Input: part model. Units: mm. Frame: model coordinates. Face numbers are marked on the shaded views. Round coordinates to 2 decimals unless told otherwise and drop trailing zeros. Write each loop counter-clockwise with the first axis right and the second up, starting at its lowest first coordinate (ties: lowest second). Pieces come first, ordered by that corner, then holes. Notation, with made-up numbers: M 89.5,-16.75 L 99.5,-16.75 A28 ccw 99.5,14.25 Z; hole C -15,-17.75 d6. An arc over 180 degrees is marked long. Answer as CSV lines item,"result". Start each with the question number.
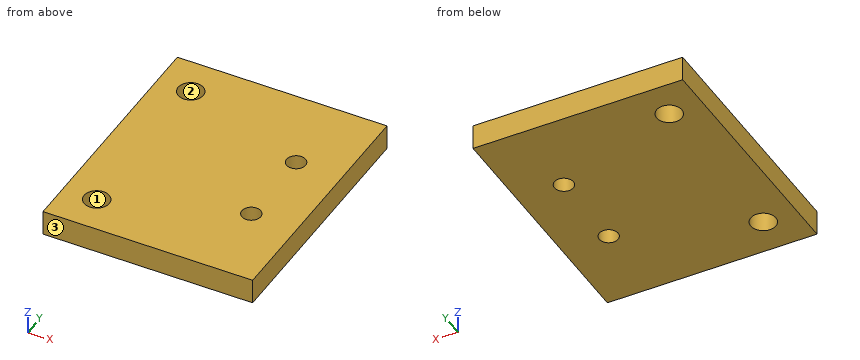
Autodesk Inventor part; units mm, degrees
ref_plane "YZ Plane" through (0, 0, 0) normal (1, 0, 0) x (0, 1, 0)
ref_plane "XZ Plane" through (0, 0, 0) normal (0, 1, 0) x (-1, 0, 0)
ref_plane "XY Plane" through (0, 0, 0) normal (0, 0, 1) x (1, 0, 0)
sketch "Sketch1" plane through (0, 0, 0) normal (0, 0, 1) x (1, 0, 0)
  line L0 (0, 0) -> (50, 0)
  line L1 (50, 0) -> (50, -60)
  line L2 (50, -60) -> (0, -60)
  line L3 (0, -60) -> (0, 0)
  circle A0 centre (8, -51) radius 3
  circle A1 centre (8, -9) radius 3
  line L4 (8, -51) -> (8, -9)
  circle A2 centre (39, -40) radius 2.25
  circle A3 centre (39, -20) radius 2.25
  line L5 (39, -40) -> (39, -20)
  dimension "d0" = 50
  dimension "d3" = 60
  dimension "d4" = 6
  dimension "d5" = 6
  dimension "d6" = 42
  dimension "d7" = 8
  dimension "d8" = 9
  dimension "d9" = 4.5
  dimension "d10" = 4.5
  dimension "d11" = 20
  dimension "d12" = 11
  dimension "d13" = 20
extrude "Extrusion1" add sketch "Sketch1" along normal blind 6
equation "\"d8\" = -0.5 * d6 + 0.5 * d3"
equation "\"d13\" = -0.5 * d11 + 0.5 * d3"
properties part number "plateencoder" material "PMMA Plastic"
Item 1: Line query: line 1 (Y direction, x = 8, z = 1.75); line 2 (Y direction, x = 39, z = 2.05); line 3 (X direction, y = -51, z = 5.65). Output: solid intervals per line, ascending. Write a range as [from, to].
Item 2: Cut plane C-C, the plane z = 5.15. Return loops of the section in (x, y), plus the area to 3 significant figures.
Item 3: Cut plane D-D, the plane x = 39. Return loops of the section in (y, z), plus the area to 3 significant figures.
Item 4: Cut plane B-B, the plane x = 8. Return loops of the section in (y, z), plus the area to 3 significant figures.
Item 5: Draft query along X for the marked faces 1, 2 and 3. Return one class per face: +X half, -X half, draft (parallel to the pull), parting line (faces both ways), or undercut.
Item 6: Cut plane A-A, the plane y = -40. Return loops of the section in (x, z).
Results list:
1,line 1,"[-60, -54], [-48, -12], [-6, 0]"
1,line 2,"[-60, -42.25], [-37.75, -22.25], [-17.75, 0]"
1,line 3,"[0, 5], [11, 50]"
2,outline,"M 0,-60 L 50,-60 L 50,0 L 0,0 Z; hole C 8,-51 d6; hole C 8,-9 d6; hole C 39,-40 d4.5; hole C 39,-20 d4.5"
2,area,"2,910 mm²"
3,outline,"M -60,0 L -42.25,0 L -42.25,6 L -60,6 Z; M -37.75,0 L -22.25,0 L -22.25,6 L -37.75,6 Z; M -17.75,0 L 0,0 L 0,6 L -17.75,6 Z"
3,area,"306 mm²"
4,outline,"M -60,0 L -54,0 L -54,6 L -60,6 Z; M -48,0 L -12,0 L -12,6 L -48,6 Z; M -6,0 L 0,0 L 0,6 L -6,6 Z"
4,area,"288 mm²"
5,face 1,"undercut"
5,face 2,"undercut"
5,face 3,"draft"
6,outline,"M 0,0 L 36.75,0 L 36.75,6 L 0,6 Z; M 41.25,0 L 50,0 L 50,6 L 41.25,6 Z"
